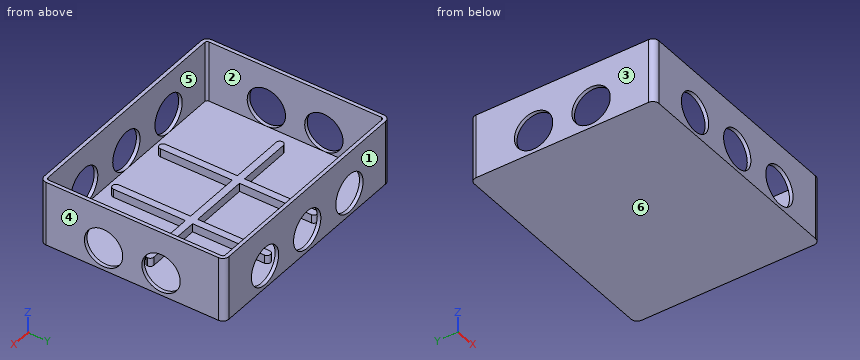
from build123d import *

# Parameters (mm, degrees)
F1_DEPTH = 54
F2_T     = -3
F3_R     = 16
F4_DEPTH = 154.001
F5_R     = 16
F6_DEPTH = 194.001
F7_W     = 6
F7_H     = 6
F7_W_2   = 49
F8_DEPTH = 7


with BuildPart() as f1:
    # F0 (on Top) → F1 (new body)
    with BuildSketch(Plane.XY):
        with BuildLine():
            ThreePointArc((97, 72), (95.5355339059, 75.5355339059), (92, 77))
            Line((92, 77), (-92, 77))
            ThreePointArc((-92, 77), (-95.5355339059, 75.5355339059), (-97, 72))
            Line((-97, 72), (-97, -72))
            ThreePointArc((-97, -72), (-95.5355339059, -75.5355339059), (-92, -77))
            Line((-92, -77), (92, -77))
            ThreePointArc((92, -77), (95.5355339059, -75.5355339059), (97, -72))
            Line((97, -72), (97, 72))
        make_face()
    extrude(amount=F1_DEPTH)

    # F2
    f2_openings = [f1.faces().sort_by_distance(p)[0] for p in [
        (0, 0, 54),
    ]]
    offset(amount=F2_T, openings=f2_openings)

    # F3 (on face) → F4 (cut, through all)
    with BuildSketch(Plane.XZ.offset(77)):
        with Locations((-49.5, 19)):
            Circle(F3_R)
        with Locations((0, 19)):
            Circle(F3_R)
        with Locations((49.5, 19)):
            Circle(F3_R)
    extrude(amount=-F4_DEPTH, mode=Mode.SUBTRACT)

    # F5 (on face) → F6 (cut, through all)
    with BuildSketch(Plane.YZ.offset(97)):
        with Locations((-24, 19)):
            Circle(F5_R)
        with Locations((24, 19)):
            Circle(F5_R)
    extrude(amount=-F6_DEPTH, mode=Mode.SUBTRACT)

    # F7 (on face) → F8 (join)
    with BuildSketch(Plane.XY.offset(3)):
        with BuildLine():
            ThreePointArc((-30.5, 62.9770308733), (-27.5, 59.9770308733), (-24.5, 62.9770308733))
            ThreePointArc((-24.5, 62.9770308733), (-27.5, 65.9770308733), (-30.5, 62.9770308733))
        make_face()
        with BuildLine():
            Line((-24.5, 3), (-24.5, 62.9770308733))
            ThreePointArc((-24.5, 62.9770308733), (-27.5, 59.9770308733), (-30.5, 62.9770308733))
            Line((-30.5, 62.9770308733), (-30.5, 3))
            Line((-30.5, 3), (-24.5, 3))
        make_face()
        with Locations((-27.5, 0)):
            Rectangle(F7_W, F7_H)
        Rectangle(F7_W_2, F7_H)
        with BuildLine():
            Line((-30.5, -3), (-30.5, 3))
            Line((-30.5, 3), (-75.992539525, 3))
            ThreePointArc((-75.992539525, 3), (-73.8712191815, 2.1213203436), (-72.992539525, 0))
            ThreePointArc((-72.992539525, 0), (-73.8712191815, -2.1213203436), (-75.992539525, -3))
            Line((-75.992539525, -3), (-30.5, -3))
        make_face()
        with Locations((27.5, 0)):
            Rectangle(F7_W, F7_H)
        with BuildLine():
            Line((24.5, 62.9770308733), (24.5, 3))
            Line((24.5, 3), (30.5, 3))
            Line((30.5, 3), (30.5, 62.9770308733))
            ThreePointArc((30.5, 62.9770308733), (27.5, 59.9770308733), (24.5, 62.9770308733))
        make_face()
        with BuildLine():
            Line((-24.5, -62.9770308733), (-24.5, -3))
            Line((-24.5, -3), (-30.5, -3))
            Line((-30.5, -3), (-30.5, -62.9770308733))
            ThreePointArc((-30.5, -62.9770308733), (-27.5, -59.9770308733), (-24.5, -62.9770308733))
        make_face()
        with BuildLine():
            ThreePointArc((-72.992539525, 0), (-73.8712191815, 2.1213203436), (-75.992539525, 3))
            ThreePointArc((-75.992539525, 3), (-78.992539525, 0), (-75.992539525, -3))
            ThreePointArc((-75.992539525, -3), (-73.8712191815, -2.1213203436), (-72.992539525, 0))
        make_face()
        with BuildLine():
            Line((30.5, -3), (24.5, -3))
            Line((24.5, -3), (24.5, -62.9770308733))
            ThreePointArc((24.5, -62.9770308733), (27.5, -59.9770308733), (30.5, -62.9770308733))
            Line((30.5, -62.9770308733), (30.5, -3))
        make_face()
        with BuildLine():
            ThreePointArc((30.5, 62.9770308733), (27.5, 65.9770308733), (24.5, 62.9770308733))
            ThreePointArc((24.5, 62.9770308733), (27.5, 59.9770308733), (30.5, 62.9770308733))
        make_face()
        with BuildLine():
            Line((75.992539525, 3), (30.5, 3))
            Line((30.5, 3), (30.5, -3))
            Line((30.5, -3), (75.992539525, -3))
            ThreePointArc((75.992539525, -3), (72.992539525, 0), (75.992539525, 3))
        make_face()
        with BuildLine():
            ThreePointArc((-30.5, -62.9770308733), (-27.5, -65.9770308733), (-24.5, -62.9770308733))
            ThreePointArc((-24.5, -62.9770308733), (-27.5, -59.9770308733), (-30.5, -62.9770308733))
        make_face()
        with BuildLine():
            ThreePointArc((30.5, -62.9770308733), (27.5, -59.9770308733), (24.5, -62.9770308733))
            ThreePointArc((24.5, -62.9770308733), (27.5, -65.9770308733), (30.5, -62.9770308733))
        make_face()
        with BuildLine():
            ThreePointArc((78.992539525, 0), (78.1138598686, 2.1213203436), (75.992539525, 3))
            ThreePointArc((75.992539525, 3), (72.992539525, 0), (75.992539525, -3))
            ThreePointArc((75.992539525, -3), (78.1138598686, -2.1213203436), (78.992539525, 0))
        make_face()
    extrude(amount=F8_DEPTH)


solid = f1.part
Geometry: final body of the model. Coordinates: model frame, mm. Face numbers are marked on the shaded views. A direction names the side the tool comes from. Give positions to 0.01 mm unless a question says otherwise; leave off trailing zeros. Write each loop counter-clockwise with the first axis right and the second up, starting at its lowest first coordinate (ties: lowest second). Pieces come first, ordered by that corner, then holes. Notation, with made-up numbers: (-21.75, 64) - (21.25, 64) arc R21 cw to (21.25, 82) - close; hole circle Ø5 at (64, 80.25). An arc over 180 degrees is marked (long way). Return JSON: item names as keys, results as strings. Group by question number.
1) First-contact query: P1, Ø8, axis at x = -66.5, y = -5, coming from the -Z side; P2, Ø6, axis at x = 74.5, y = 50, coming from the +Z side; P3, Ø2, axis at y = -30, z = 5.5, coming from the +X side; P4, Ø3.5, axis at y = -21, z = 5.5, coming from the -X side. Flat tips, straight axial feed; report the tip coordinate or a pass-through.
2) Section C-C on y = 15.5. Return the cut outline in (x, z).
3) Section A-A on x = -27.5. Return the cut outline in (y, z).
4) Section D-D on y = 49. Return the cut outline in (x, z), plus the area to 3 significant figures.
5) Mould query, pull axis X, two halves, no side actions, for the marked faces 3, 4, 5 and 6. Classes: released by +X, released by -X, zero draft, split by the parting line, or undercut.
6) Section B-B on z = 46.5. Return the cut outline in (x, y), plus the area to 3 significant figures.
7) Line query: line 1 (X direction, y = 53, z = 49); line 2 (Y direction, x = 37, z = 42); line 3 (Y direction, x = 95, z = 19). Output: solid intervals per line, ascending.
8) Set-up query: the marked faces 1 and 2. Return all of +Z, -Z, +X, -X, +Y, -Y with unobstructed straight access to the full face (end or side cutting, diameter ignored); none if empty.
Filled in:
{
 "1": {"P1": "stops at z = 0", "P2": "stops at z = 3", "P3": "stops at x = 30.5", "P4": "stops at x = -30.5"},
 "2": {"outline": "(-97, 0) - (97, 0) - (97, 5.44) - (94, 5.44) - (94, 3) - (30.5, 3) - (30.5, 10) - (24.5, 10) - (24.5, 3) - (-24.5, 3) - (-24.5, 10) - (-30.5, 10) - (-30.5, 3) - (-94, 3) - (-94, 5.44) - (-97, 5.44) - close; (-97, 32.56) - (-94, 32.56) - (-94, 54) - (-97, 54) - close; (94, 32.56) - (97, 32.56) - (97, 54) - (94, 54) - close"},
 "3": {"outline": "(-77, 0) - (77, 0) - (77, 54) - (74, 54) - (74, 3) - (65.98, 3) - (65.98, 10) - (-65.98, 10) - (-65.98, 3) - (-74, 3) - (-74, 54) - (-77, 54) - close"},
 "4": {"outline": "(-97, 0) - (97, 0) - (97, 54) - (94, 54) - (94, 3) - (30.5, 3) - (30.5, 10) - (24.5, 10) - (24.5, 3) - (-24.5, 3) - (-24.5, 10) - (-30.5, 10) - (-30.5, 3) - (-94, 3) - (-94, 54) - (-97, 54) - close", "area": "972 mm^2"},
 "5": {"face 3": "released by -X", "face 4": "released by +X", "face 5": "undercut", "face 6": "zero draft"},
 "6": {"outline": "(-97, -72) arc R5 ccw to (-92, -77) - (92, -77) arc R5 ccw to (97, -72) - (97, 72) arc R5 ccw to (92, 77) - (-92, 77) arc R5 ccw to (-97, 72) - close; hole (-94, -72) arc R2 ccw to (-92, -74) - (92, -74) arc R2 ccw to (94, -72) - (94, 72) arc R2 ccw to (92, 74) - (-92, 74) arc R2 ccw to (-94, 72) - close", "area": "2,030 mm^2"},
 "7": {"line 1": "x = -97 to -94, 94 to 97", "line 2": "y = -77 to -74, 74 to 77", "line 3": "y = -76 to -40, -8 to 8, 40 to 76"},
 "8": {"face 1": "+Z, -Z, +X, -X, +Y", "face 2": "+Z"}
}
